from build123d import *

# Parameters (mm, degrees)
SKETCH1_W           = 45
SKETCH1_H           = 26
BOSS_EXTRUDE2_DEPTH = 9.5
SHELL2_T            = -1
SKETCH2_R           = 4
SKETCH2_W           = 6
SKETCH2_H           = 12.5
CUT_EXTRUDE1_DEPTH  = 9.5
SKETCH3_W           = 15
SKETCH3_H           = 6
BOSS_EXTRUDE4_DEPTH = 3
SKETCH4_R           = 1.6
CUT_EXTRUDE2_DEPTH  = 9
SKETCH5_R           = 1.75
CUT_EXTRUDE3_DEPTH  = 9


with BuildPart() as part:
    # Sketch1 → Boss-Extrude2 (new body)
    with BuildSketch(Plane.XY):
        Rectangle(SKETCH1_W, SKETCH1_H)
    extrude(amount=BOSS_EXTRUDE2_DEPTH)

    # Shell2
    shell2_openings = [part.faces().sort_by_distance(p)[0] for p in [
        (0, 0, 0),
    ]]
    offset(amount=SHELL2_T, openings=shell2_openings, kind=Kind.INTERSECTION)

    # Sketch2 → Cut-Extrude1 (cut)
    with BuildSketch(Plane(origin=(0, 0, 8.5), x_dir=(-1, 0, 0), z_dir=(0, 0, -1))):
        with Locations((13.5, 0)):
            Circle(SKETCH2_R)
        with Locations((-16.6, 0)):
            Rectangle(SKETCH2_W, SKETCH2_H)
    extrude(amount=-CUT_EXTRUDE1_DEPTH, mode=Mode.SUBTRACT)

    # Sketch3 → Boss-Extrude4 (add)
    with BuildSketch(Plane(origin=(0, 0, 0), x_dir=(-1, 0, 0), z_dir=(0, 0, -1))):
        with Locations((7.5, 16)):
            Rectangle(SKETCH3_W, SKETCH3_H)
        with Locations((7.5, -16)):
            Rectangle(SKETCH3_W, SKETCH3_H)
    extrude(amount=-BOSS_EXTRUDE4_DEPTH)

    # Sketch4 → Cut-Extrude2 (cut)
    with BuildSketch(Plane.XY.offset(3)):
        with Locations((-8.674253425, -16.212560211)):
            Circle(SKETCH4_R)
    extrude(amount=-CUT_EXTRUDE2_DEPTH, mode=Mode.SUBTRACT)

    # Sketch5 → Cut-Extrude3 (cut)
    with BuildSketch(Plane.XY.offset(3)):
        with Locations((-9.262710237, 15.798173241)):
            Circle(SKETCH5_R)
    extrude(amount=-CUT_EXTRUDE3_DEPTH, mode=Mode.SUBTRACT)


solid = part.part
Part model, mm, in its own coordinate system. A direction names the side the tool comes from. Give positions to 0.01 mm unless a question says otherwise; leave off trailing zeros. Loops run counter-clockwise (first coordinate to the right, second up) from the corner with the lowest first, then second, coordinate; pieces in that order, holes last. Notation, with made-up numbers: M 61.5,81 L 105.5,81 A20 ccw 105.5,88 Z; hole C 65,-1 d10. An arc over 180 degrees is marked long. Put each result on its own line as item: value. Start each with the question number.
1) Probe probe 1 along X at (y, z) = (-0.5, 3.5); probe 2 along Y at (x, z) = (-13.5, 9.2); probe 3 along Y at (x, z) = (13, 1). List the from-to ranges inside material, lowest first.
2) Flat gauge pins, fed straight in: pin 1 (1.8 mm diameter, centred on x = -7, y = -16.5, fed in from +Z); pin 2 (12 mm diameter, centred on x = 2.5, y = -7, fed in from -Z); pin 3 (3 mm diameter, centred on x = -9.26, y = 15.8, fed in from -Z); pin 4 (5 mm diameter, centred on x = 6, z = 5.5, fed in from +Y). Where does each tip first touch, or does it go through?
3) 3-axis set-ups, long thin cutter, end or side, ignore diameter. For faces 1 (the flat face through (-7, -15, 3)), 2 (the flat face through (-15, 16, 1)), 3 (the flat face through (0, -12, 4)), 4 (the flat face through (19.6, 0, 9)): which of +Z, -Z, +X, -X, +Y, -Y reach the whole face in a straight line?
4) Saw through at A-A (y = 0). List the corners of the cut face in (x, z), then the cut area to 3 significant figures.
5) Saw through at C-C (z = 5.5). List the corners of the cut face in (x, y).
6) Saw through at D-D (y = 15). List the corners of the cut face in (x, z).
7) Saw through at B-B (x = -13.5). List the corners of the cut face in (y, z).
8) Pull direction Y, two halves, no side cores. Call faces 5 (the flat face through (17, -6.25, 9)), 6 (the flat face through (-7, 19, 1)), 7 (the flat face through (0, -16, 1)): +Y half, -Y half, draft (parallel to the pull), parting line (faces both ways), or undercut.
Numbers:
1. probe 1: -22.5 to -21.5, 21.5 to 22.5
1. probe 2: -13 to -4, 4 to 13
1. probe 3: -13 to -12, 12 to 13
2. pin 1: z = 3
2. pin 2: z = 0
2. pin 3: through
2. pin 4: y = 13
3. face 1: +Z, +X, -X, -Y
3. face 2: +Z, -Z, -X, +Y
3. face 3: -Z
3. face 4: +Z, -Z
4. outline: M -22.5,0 L -21.5,0 L -21.5,8.5 L -17.5,8.5 L -17.5,9.5 L -22.5,9.5 Z; M -9.5,8.5 L 13.6,8.5 L 13.6,9.5 L -9.5,9.5 Z; M 19.6,8.5 L 21.5,8.5 L 21.5,0 L 22.5,0 L 22.5,9.5 L 19.6,9.5 Z
4. area: 48.0 mm^2
5. outline: M -22.5,-13 L 22.5,-13 L 22.5,13 L -22.5,13 Z; hole M -21.5,-12 L 21.5,-12 L 21.5,12 L -21.5,12 Z
6. outline: M -15,0 L -10.82,0 L -10.82,3 L -15,3 Z; M -7.71,0 L 0,0 L 0,3 L -7.71,3 Z
7. outline: M -19,0 L -12,0 L -12,8.5 L -4,8.5 L -4,9.5 L -13,9.5 L -13,3 L -19,3 Z; M 4,8.5 L 12,8.5 L 12,0 L 19,0 L 19,3 L 13,3 L 13,9.5 L 4,9.5 Z
8. face 5: undercut
8. face 6: +Y half
8. face 7: draft
